```python
from build123d import *

# Parameters (mm, degrees)
SKETCH1_R           = 18.5
BOSS_EXTRUDE1_DEPTH = 3
SKETCH2_R           = 18
SKETCH2_R_2         = 13
CUT_EXTRUDE1_DEPTH  = 1.5
SCALE1_SCALE        = 0.8


with BuildPart() as part:
    # Sketch1 → Boss-Extrude1 (new body)
    with BuildSketch(Plane(origin=(0, 0, 0), x_dir=(1, 0, 0), z_dir=(0, 1, 0))):
        with Locations(Location((0, 0, 0), (0, 0, 270))):
            Circle(SKETCH1_R)
    extrude(amount=BOSS_EXTRUDE1_DEPTH)

    # Sketch2 → Cut-Extrude1 (cut)
    with BuildSketch(Plane(origin=(0, 3, 0), x_dir=(1, 0, 0), z_dir=(0, 1, 0))):
        with Locations(Location((0, 0, 0), (0, 0, 270))):
            Circle(SKETCH2_R)
        with Locations(Location((0, 0, 0), (0, 0, 270))):
            Circle(SKETCH2_R_2, mode=Mode.SUBTRACT)
    extrude(amount=-CUT_EXTRUDE1_DEPTH, mode=Mode.SUBTRACT)


with BuildPart() as part_1:
    # Scale1: scaled about (0, 1.280453258, 0)
    add(part.part.scale(SCALE1_SCALE).moved(Location((0, 0.256090652, 0))))


solid = part_1.part
```
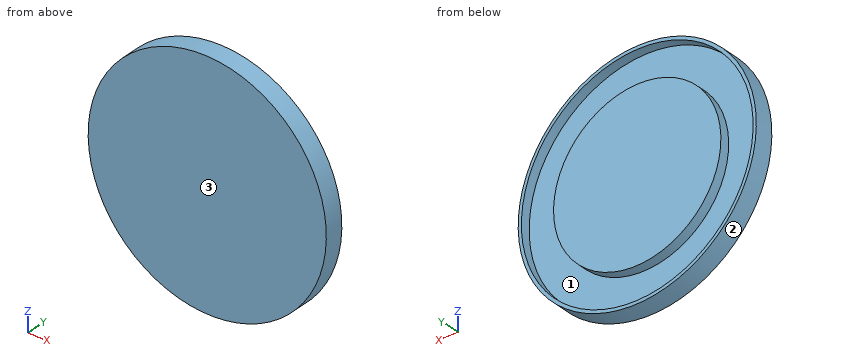
Here's how the part is built. I have some questions about the finished solid (model axes, mm). Face numbers are marked on the shaded views. Round coordinates to 2 decimals unless told otherwise and drop trailing zeros. Write each loop counter-clockwise with the first axis right and the second up, starting at its lowest first coordinate (ties: lowest second). Pieces come first, ordered by that corner, then holes.
Q1. If we mould it in two halves opening along Z, with no side actions, what happens to the marked faces 1, 2 and 3? For each: +Z half, -Z half, draft (parallel to the pull), parting line (faces both ways), or undercut.
Q2. If we section it at B-B on x = 0: Write out the boundary of the cut face in (y, z), plus the area to 3 significant figures.
Q3. If we section it at C-C on z = 0: Write out the boundary of the cut face in (x, y).
Q4. If we section it at D-D on z = 11: Write out the boundary of the cut face in (x, y), plus the area to 3 significant figures.
Q5. If we section it at A-A on y = 1.9: Write out the boundary of the cut face in (x, z).
Q6. Please list where these lines run through material, in increasing order: probe 1 along X at (y, z) = (2.15, 0); probe 2 along Z at (x, y) = (-0.5, 2.35); probe 3 along X at (y, z) = (2.55, -9).
Answer below:
1. face 1: undercut
1. face 2: parting line
1. face 3: draft
2. outline: (0.26, -14.8) - (2.66, -14.8) - (2.66, -14.4) - (1.46, -14.4) - (1.46, -10.4) - (2.66, -10.4) - (2.66, 10.4) - (1.46, 10.4) - (1.46, 14.4) - (2.66, 14.4) - (2.66, 14.8) - (0.26, 14.8) - close
2. area: 61.4 mm2
3. outline: (-14.8, 0.26) - (14.8, 0.26) - (14.8, 2.66) - (14.4, 2.66) - (14.4, 1.46) - (10.4, 1.46) - (10.4, 2.66) - (-10.4, 2.66) - (-10.4, 1.46) - (-14.4, 1.46) - (-14.4, 2.66) - (-14.8, 2.66) - close
4. outline: (-9.9, 0.26) - (9.9, 0.26) - (9.9, 2.66) - (9.29, 2.66) - (9.29, 1.46) - (-9.29, 1.46) - (-9.29, 2.66) - (-9.9, 2.66) - close
4. area: 25.2 mm2
5. outline: circle Ø29.6 at (0, 0); circle Ø20.8 at (0, 0); hole circle Ø28.8 at (0, 0)
6. probe 1: x = -14.8 to -14.4, -10.4 to 10.4, 14.4 to 14.8
6. probe 2: z = -14.79 to -14.39, -10.39 to 10.39, 14.39 to 14.79
6. probe 3: x = -11.75 to -11.24, -5.21 to 5.21, 11.24 to 11.75
